Autodesk Inventor part; units mm, degrees
ref_plane "YZ Plane" through (0, 0, 0) normal (1, 0, 0) x (0, 1, 0)
ref_plane "XZ Plane" through (0, 0, 0) normal (0, 1, 0) x (-1, 0, 0)
ref_plane "XY Plane" through (0, 0, 0) normal (0, 0, 1) x (1, 0, 0)
sketch "Sketch1" plane through (0, 0, 0) normal (0, 1, 0) x (-1, 0, 0)
  line L0 (0, 0) -> (127, 0)
  line L1 (127, 0) -> (127, -127)
  line L2 (127, -127) -> (0, -127)
  line L3 (0, -127) -> (0, 0)
  line L4 (123.825, 0) -> (127, 0)
  line L5 (127, 0) -> (127, -33.615)
  line L6 (127, -33.615) -> (123.825, -33.615)
  line L7 (123.825, -33.615) -> (123.825, 0)
  line L8 (123.825, -33.615) -> (70.363, -33.615)
  line L9 (70.363, -33.615) -> (70.363, -36.79)
  line L10 (70.363, -36.79) -> (127, -36.79)
  line L11 (70.363, -36.79) -> (67.188, -36.79)
  line L12 (67.188, -36.79) -> (67.188, 0)
  line L13 (67.188, 0) -> (70.363, 0)
  line L14 (70.363, 0) -> (70.363, -36.79)
  line L15 (127, -90.21) -> (67.188, -90.21)
  line L16 (67.188, -90.21) -> (67.188, -93.385)
  line L17 (67.188, -93.385) -> (127, -93.385)
  line L18 (127, -93.385) -> (127, -90.21)
  line L19 (127, -93.385) -> (123.825, -93.385)
  line L20 (123.825, -93.385) -> (123.825, -127)
  line L21 (123.825, -127) -> (127, -127)
  line L22 (127, -127) -> (127, -93.385)
  line L23 (25.4, 0) -> (6.35, 0)
  line L24 (25.4, -127) -> (6.35, -127)
  line L25 (67.188, -90.21) -> (70.363, -90.21)
  line L26 (70.363, -90.21) -> (70.363, -127)
  line L27 (70.363, -127) -> (67.188, -127)
  line L28 (67.188, -127) -> (67.188, -90.21)
  line L29 (67.188, -3.175) -> (70.363, -3.175)
  line L30 (70.363, -3.175) -> (70.363, -33.615)
  line L31 (70.363, -33.615) -> (67.188, -33.615)
  line L32 (67.188, -33.615) -> (67.188, -3.175)
  line L33 (73.538, -33.615) -> (123.825, -33.615)
  line L34 (123.825, -33.615) -> (123.825, -36.79)
  line L35 (123.825, -36.79) -> (73.538, -36.79)
  line L36 (127, -3.175) -> (123.825, -3.175)
  line L37 (123.825, -3.175) -> (123.825, -30.44)
  line L38 (123.825, -30.44) -> (127, -30.44)
  line L39 (127, -30.44) -> (127, -3.175)
  line L40 (123.825, -90.21) -> (81.7068, -90.21)
  line L41 (81.7068, -93.385) -> (123.825, -93.385)
  line L42 (123.825, -93.385) -> (123.825, -90.21)
  line L43 (123.825, -96.56) -> (127, -96.56)
  line L44 (127, -96.56) -> (127, -123.825)
  line L45 (127, -123.825) -> (123.825, -123.825)
  line L46 (123.825, -123.825) -> (123.825, -96.56)
  line L47 (70.363, -96.56) -> (67.188, -96.56)
  line L48 (67.188, -96.56) -> (67.188, -123.825)
  line L49 (67.188, -123.825) -> (70.363, -123.825)
  line L50 (70.363, -123.825) -> (70.363, -96.56)
  line L51 (70.363, -30.44) -> (67.188, -30.44)
  line L52 (22.225, 0) -> (9.525, 0)
  line L53 (9.525, -127) -> (22.225, -127)
  line L54 (127, 0) -> (130.175, 0)
  line L55 (130.175, 0) -> (130.175, -127)
  line L56 (130.175, -127) -> (127, -127)
  line L57 (127, -127) -> (127, 0)
  line L58 (3.175, 0) -> (0, 0)
  line L59 (0, 0) -> (0, -127)
  line L60 (0, -127) -> (3.175, -127)
  line L61 (3.175, -127) -> (3.175, 0)
  line L62 (62.987, 0) -> (62.987, -33.6042)
  line L63 (62.987, -33.6042) -> (59.812, -33.6042)
  line L64 (59.812, -33.6042) -> (59.812, -4.3263)
  line L65 (59.812, -33.6042) -> (6.35, -33.6042)
  line L66 (6.35, -33.6042) -> (6.35, -36.7792)
  line L67 (6.35, -36.7792) -> (62.987, -36.7792)
  line L68 (6.35, -36.7792) -> (3.175, -36.7792)
  line L69 (3.175, -36.7792) -> (3.175, -2.1822)
  line L70 (6.35, 0) -> (6.35, -36.7792)
  line L71 (3.175, -3.175) -> (6.35, -3.175)
  line L72 (6.35, -3.175) -> (6.35, -33.6042)
  line L73 (6.35, -33.6042) -> (3.175, -33.6042)
  line L74 (3.175, -33.6042) -> (3.175, -3.175)
  line L75 (59.812, -33.6042) -> (59.812, -36.7792)
  line L76 (62.987, -3.175) -> (59.812, -3.175)
  line L77 (59.812, -3.175) -> (59.812, -30.4292)
  line L78 (59.812, -30.4292) -> (62.987, -30.4292)
  line L79 (62.987, -30.4292) -> (62.987, -3.175)
  line L80 (6.35, -30.4292) -> (3.175, -30.4292)
  line L81 (62.987, -36.7792) -> (62.987, 0)
  line L82 (59.812, -3.175) -> (59.812, 0)
  line L83 (62.992, -127) -> (59.817, -127)
  line L84 (59.817, -127) -> (59.817, -90.2208)
  line L85 (59.817, -90.2208) -> (62.992, -90.2208)
  line L86 (62.992, -90.2208) -> (62.992, -127)
  line L87 (62.992, -93.3958) -> (3.175, -93.3958)
  line L88 (3.175, -93.3958) -> (3.175, -90.2208)
  line L89 (3.175, -90.2208) -> (62.992, -90.2208)
  line L90 (62.992, -90.2208) -> (62.992, -93.3958)
  line L91 (6.35, -90.2208) -> (3.175, -90.2208)
  line L92 (3.175, -90.2208) -> (3.175, -127)
  line L93 (3.175, -127) -> (6.35, -127)
  line L94 (6.35, -127) -> (6.35, -90.2208)
  line L95 (6.35, -123.825) -> (3.175, -123.825)
  line L96 (3.175, -123.825) -> (3.175, -96.5708)
  line L97 (3.175, -96.5708) -> (6.35, -96.5708)
  line L98 (6.35, -96.5708) -> (6.35, -123.825)
  line L99 (62.992, -123.825) -> (59.817, -123.825)
  line L100 (59.817, -123.825) -> (59.817, -96.5708)
  line L101 (59.817, -96.5708) -> (62.992, -96.5708)
  line L102 (62.992, -96.5708) -> (62.992, -123.825)
  point P0 (97.094, -33.615)
  point P1 (123.825, -110.1925)
  point P2 (123.825, -16.8075)
  point P3 (125.4125, 0)
  point P4 (125.4125, -3.175)
  point P5 (125.4125, -33.615)
  point P6 (70.363, -35.2025)
  point P7 (68.7755, -36.79)
  point P8 (68.7755, -33.615)
  point P9 (68.7755, 0)
  point P10 (68.7755, -3.175)
  point P11 (68.7755, -127)
  point P12 (68.7755, -123.825)
  point P13 (70.363, -93.385)
  point P14 (70.363, -30.44)
  point P15 (127, -96.56)
  point P16 (127, -30.44)
  point P17 (123.825, -33.615)
  point P18 (67.188, -96.56)
  point P19 (127, -93.385)
  point P20 (33.081, -33.6042)
  point P21 (59.812, -18.9652)
  point P22 (61.3995, -3.175)
  point P23 (61.3995, -33.6042)
  point P24 (6.35, -35.1917)
  point P25 (4.7625, -36.7792)
  point P26 (4.7625, -33.6042)
  point P27 (4.7625, -3.175)
  point P28 (59.817, -93.3958)
  point P29 (6.35, -93.3958)
  point P30 (3.175, -3.175)
  dimension "d0" = 127
  dimension "d2" = 127
  dimension "d5" = 33.615
  dimension "d6" = 33.615
  dimension "d7" = 53.462
  dimension "d8" = 53.462
  dimension "d9" = 3.175
  dimension "d10" = 3.175
  dimension "d11" = 3.175
  dimension "d12" = 3.175
  dimension "d13" = 3.175
  dimension "d14" = 3.175
  dimension "d28" = 3.175
  dimension "d29" = 3.175
  dimension "d30" = 3.175
  dimension "d32" = 3.175
  dimension "d33" = 3.175
  dimension "d34" = 3.175
  dimension "d35" = 3.175
  dimension "d36" = 3.175
  dimension "d37" = 3.175
  dimension "d38" = 3.175
  dimension "d57" = 3.175
  dimension "d58" = 3.175
  dimension "d90" = 53.462
  dimension "d91" = 3.175
  dimension "d92" = 3.175
  dimension "d93" = 3.175
  dimension "d94" = 3.175
  dimension "d96" = 3.175
  dimension "d97" = 3.175
  dimension "d98" = 0
  dimension "d99" = 3.175
  dimension "d100" = 3.175
  dimension "d101" = 33.6042
  dimension "d102" = 33.6042
  dimension "d103" = 53.467
  dimension "d104" = 0
  dimension "d105" = 0
  dimension "d106" = 0
  dimension "d107" = 3.175
  dimension "d108" = 3.175
  dimension "d109" = 3.175
  dimension "d110" = 3.175
  dimension "d111" = 3.175
  dimension "d112" = 3.175
  dimension "d113" = 3.175
extrude "Extrusion1" add sketch "Sketch1" along normal blind 3.175 contours L0 L61 L2 L3 | L0 L70 L71 L61 | L0 L82 L77 L64 L65 L70 | L61 L95 L94 L2 | L94 L87 L84 L2 | L70 L73 L61 L80 | L61 L87 L94 L97 | L66 L68 L61 L73 | L61 L89 L94 L87 | L0 L62 L76 L82 | L64 L78 L62 L63 | L63 L81 L67 L75 | L67 L81 L62 L0 L12 L11 L10 L1 L15 L16 L28 L2 L86 L85 L89 L61 L68 | L84 L99 L86 L2 | L87 L86 L101 L84 | L84 L85 L86 L87 | L0 L14 L29 L12 | L0 L7 L8 L14 | L28 L49 L26 L2 | L0 L1 L36 L7 | L51 L14 L31 L12 | L26 L17 L20 L2 | L54 L55 L56 L1 | L31 L9 L11 L12 | L20 L45 L1 L2 | L28 L17 L26 L47 | L38 L1 L6 L7 | L16 L15 L26 L17 | L6 L1 L10 L34 | L20 L17 L1 L43 | L42 L15 L1 L17
equation "\"d3\" = d41"
properties part number "top"
Build history of the part. All positions in model axes, mm. Round coordinates to 2 decimals unless told otherwise and drop trailing zeros. Order: outer loops, then holes, each group sorted by start corner. A loop starts at its lowest first (then second) coordinate and runs counter-clockwise, first axis right, second up. Notation, with made-up numbers: (39, -38) -> (89, -38) arc R13 cw to (89, -26) -> close; hole circle Ø8 at (46.5, 35). An arc over 180 degrees is marked (long way). Answer in a Markdown table with one row per item.
1) Band-saw the part on B-B on z = -114. Give the cut face in (x, y) (3 decimals), and give its area (3 significant figures).
Values:
| item | result |
|---|---|
| outline | (-130.175, 0) -> (-127, 0) -> (-127, 3.175) -> (-130.175, 3.175) -> close; (-123.825, 0) -> (-70.363, 0) -> (-70.363, 3.175) -> (-123.825, 3.175) -> close; (-67.188, 0) -> (-62.992, 0) -> (-62.992, 3.175) -> (-67.188, 3.175) -> close; (-59.817, 0) -> (-6.35, 0) -> (-6.35, 3.175) -> (-59.817, 3.175) -> close; (-3.175, 0) -> (0, 0) -> (0, 3.175) -> (-3.175, 3.175) -> close |
| area | 373 mm2 |
2) Band-saw the part on C-C on y = 0.55. Give the number of separate pieces and of enclosed holes in the cut face, and give its area (3 significant figures).
Values:
| item | result |
|---|---|
| separate pieces | 1 |
| enclosed holes | 12 |
| area | 15,200 mm2 |
3) Pin check, flat tip, straight feed: P1, Ø2, axis at x = -36, z = -19, coming from the -Y side. Stop position of the tip, or through.
Values:
| item | result |
|---|---|
| P1 | y = 0 |
4) Band-saw the part on A-A on x = -8.5. Give the cut face in (y, z) (3 decimals).
Values:
| item | result |
|---|---|
| outline | (0, -127) -> (3.175, -127) -> (3.175, -93.396) -> (0, -93.396) -> close; (0, -90.221) -> (3.175, -90.221) -> (3.175, -36.779) -> (0, -36.779) -> close; (0, -33.604) -> (3.175, -33.604) -> (3.175, 0) -> (0, 0) -> close |
5) Mould opens along Z. For faces 1 (the flat face through (-64, 3.175, -63)), 2 (the flat face through (-5, 2, -3.175)) say: released by +Z, released by -Z, zero draft, split by the parting line, or undercut.
Values:
| item | result |
|---|---|
| face 1 | zero draft |
| face 2 | undercut |
6) Wall check: L1, parallel to Z at x = -122, y = 1.6 (3 decimals); L2, parallel to X at y = 2.6, z = -26 (3 decimals). Give the ranges that are in metal, low to high.
Values:
| item | result |
|---|---|
| L1 | -127 to -93.385, -90.21 to -36.79, -33.615 to 0 |
| L2 | -130.175 to -127, -123.825 to -70.363, -67.188 to -62.987, -59.812 to -6.35, -3.175 to 0 |
